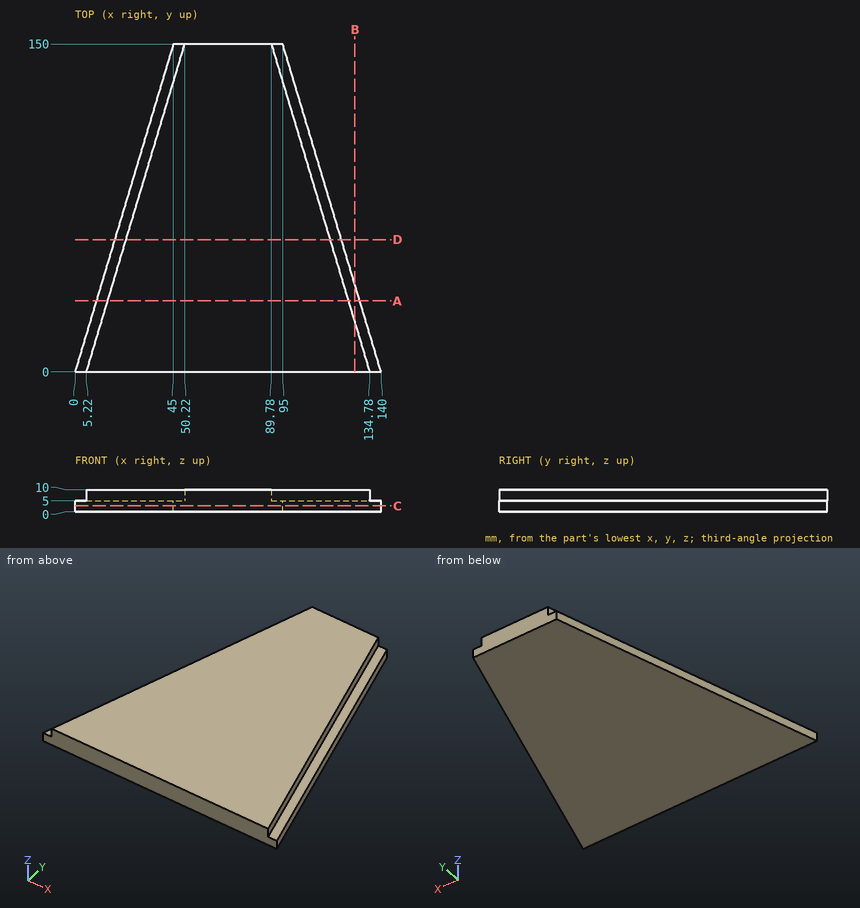
Job drawing, mm, ordinate dimensions from the low corner. One solid piece. Coordinates: 2 decimals unless noted, no trailing zeros. Order: outer loops, then holes, each group sorted by start corner. A loop starts at its lowest first (then second) coordinate and runs counter-clockwise, first axis right, second up. Notation, with made-up numbers: (46, -21) -> (52, -21) arc R31 ccw to (52, 17) -> close; hole circle Ø9 at (76.5, -38.5). An arc over 180 degrees is marked (long way). Return JSON: item names as keys, results as strings. Group by question number.
Item 1: Saw through at B-B on x = 128. Write the cut outline in (y, z).
Item 2: Saw through at D-D on y = 60.5. Write the cut outline in (x, z).
Item 3: Saw through at A-A on y = 32.5. Write the cut outline in (x, z).
Item 4: Wall check: line 1 along X through (y, z) = (59, 6.5); line 2 along X through (y, z) = (67, 8.5). Give the ranges that are in metal, low to high. Write a range as [from, to].
Item 5: Flat gauge pins, fed straight in: P1, Ø4, axis at y = 27, z = 5.5, coming from the +X side; P2, Ø1.5, axis at y = 77, z = 4, coming from the +X side (3 decimals). Where does each tip first touch, or does it go through?
Item 6: Saw through at C-C on z = 2.75. Write the cut outline in (x, y).
Values found:
{
 "1": {"outline": "(0, 0) -> (40, 0) -> (40, 5) -> (22.6, 5) -> (22.6, 10) -> (0, 10) -> close"},
 "2": {"outline": "(18.15, 0) -> (121.85, 0) -> (121.85, 5) -> (116.63, 5) -> (116.63, 10) -> (23.37, 10) -> (23.37, 5) -> (18.15, 5) -> close"},
 "3": {"outline": "(9.75, 0) -> (130.25, 0) -> (130.25, 5) -> (125.03, 5) -> (125.03, 10) -> (14.97, 10) -> (14.97, 5) -> (9.75, 5) -> close"},
 "4": {"line 1": "x = [22.92, 117.08]", "line 2": "x = [25.32, 114.68]"},
 "5": {"P1": "stops at x = 132.48", "P2": "stops at x = 117.125"},
 "6": {"outline": "(0, 0) -> (140, 0) -> (95, 150) -> (45, 150) -> close"}
}
